Build history of the part. All positions in model axes, mm. A direction names the side the tool comes from. Give positions to 0.01 mm unless a question says otherwise; leave off trailing zeros. Order: outer loops, then holes, each group sorted by start corner. A loop starts at its lowest first (then second) coordinate and runs counter-clockwise, first axis right, second up. Notation, with made-up numbers: (25, 49.25) - (55, 49.25) arc R22 ccw to (55, 79.25) - close; hole circle Ø1 at (10.25, 87). An arc over 180 degrees is marked (long way). Use a Markdown table: item, result. Add a question column.
(1) Flat gauge pins, fed straight in: pin 1 (6 mm diameter, centred on y = -20, z = 23, fed in from +X); pin 2 (4 mm diameter, centred on x = 8.5, z = 6.5, fed in from +Y); pin 3 (12 mm diameter, centred on y = -15.5, z = 14, fed in from +X). Where does each tip first touch, or does it go through?
(2) Which spindle directions (+Z, -Z, +X, -X, +Y, -Y) get a long thin tool onto all of the face, cutting with end or side? Do faces 1 (the face through (17.314, 9.811, 21.731)), 2 (the face through (19, -13, 20.2)), 3 (the face through (-6.092, 27.432, 4.93)). Say none if no direction does.
(3) Slice it at C-C (y = 16.5). Write the cut outline in (x, z), then the cut area to 3 significant figures.
(4) Slice it at B-B (z = 34). Write the cut outline in (x, y).
(5) Slice it at A-A (z = 9). Write the cut outline in (x, y), then the cut area to 3 significant figures.
(6) Slice it at D-D (x = 14). Write the cut outline in (y, z).
(7) Wall check: line 1 (Y direction, x = 0, z = 6); line 2 (Y direction, x = 0, z = 34.75); line 3 (Y direction, x = 0, z = 26). Give the ranges that are in metal, low to high.
(8) Mould opens along Y. For faces 4 (the face through (-28, -21, 2)), 5 (the face through (-2.55, 22, 21)), 6 (the face through (17, -11, 38)), 7 (the face through (0, 24.95, 21)) say: +Y half, -Y half, draft (parallel to the pull), parting line (faces both ways), or undercut.
from build123d import *

# Parameters (mm, degrees)
CUT_EXTRUDE1_DEPTH = 71.512410255
SKETCH3_R          = 1.5
CUT_EXTRUDE2_DEPTH = 20
SKETCH4_W          = 5.1
SKETCH4_H          = 5.05
CUT_EXTRUDE3_DEPTH = 1.8
SKETCH6_R          = 2.55
CUT_EXTRUDE4_DEPTH = 3
SKETCH7_R          = 1.75
CUT_EXTRUDE5_DEPTH = 3
SKETCH8_OUTSIDE_W  = 110.944
SKETCH8_OUTSIDE_H  = 110.944
SKETCH8_OUTSIDE_R  = 35
CUT_EXTRUDE6_DEPTH = 71.512410255


with BuildPart() as part:
    # Sketch1 → Revolve1 (revolve)
    with BuildSketch(Plane(origin=(0, 0, 0), x_dir=(1, 0, 0), z_dir=(0, 1, 0))):
        Polygon((19.9, -38), (19.9, -5), (24.95, -5), (24.95, -10), (28.1, -10), (28.1, 0), (42, 0), (42, -5), (31.25, -5), (31.25, -30), (24.95, -30), (24.95, -38), align=None)
    revolve(axis=Axis((0, 0, 57.825795551), (0, 0, -1)))

    # Sketch2 → Cut-Extrude1 (cut, through all)
    with BuildSketch(Plane.XY.offset(38)):
        Polygon((-22.978540714, 0), (-11.489270357, -19.9), (11.489270357, -19.9), (22.978540714, 0), (11.489270357, 19.9), (-11.489270357, 19.9), align=None)
    extrude(amount=-CUT_EXTRUDE1_DEPTH, mode=Mode.SUBTRACT)

    # Sketch3 → Cut-Extrude2 (cut)
    with BuildSketch(Plane.XY.offset(38)):
        with Locations((0, 22.4)):
            Circle(SKETCH3_R)
        with Locations((19.398969045, -11.2)):
            Circle(SKETCH3_R)
        with Locations((-19.398969045, -11.2)):
            Circle(SKETCH3_R)
    extrude(amount=-CUT_EXTRUDE2_DEPTH, mode=Mode.SUBTRACT)

    # Sketch4 → Cut-Extrude3 (cut)
    with BuildSketch(Plane.XY.offset(22)):
        with Locations((0, 22.425)):
            Rectangle(SKETCH4_W, SKETCH4_H)
        Polygon((18.508905535, -7.74163522), (15.958905535, -12.15836478), (20.332333824, -14.68336478), (22.882333824, -10.26663522), align=None)
        Polygon((-15.958905535, -12.15836478), (-18.508905535, -7.74163522), (-22.882333824, -10.26663522), (-20.332333824, -14.68336478), align=None)
    extrude(amount=-CUT_EXTRUDE3_DEPTH, mode=Mode.SUBTRACT)

    # Sketch6 → Cut-Extrude4 (cut)
    with BuildSketch(Plane(origin=(0, 0, 0), x_dir=(-1, 0, 0), z_dir=(0, 0, -1))):
        with Locations((0, 38)):
            Circle(SKETCH6_R)
        with Locations((38, 0)):
            Circle(SKETCH6_R)
        with Locations((0, -38)):
            Circle(SKETCH6_R)
        with Locations((-38, 0)):
            Circle(SKETCH6_R)
    extrude(amount=-CUT_EXTRUDE4_DEPTH, mode=Mode.SUBTRACT)

    # Sketch7 → Cut-Extrude5 (cut)
    with BuildSketch(Plane(origin=(0, 0, 3), x_dir=(-1, 0, 0), z_dir=(0, 0, -1))):
        with Locations((0, 38)):
            Circle(SKETCH7_R)
        with Locations((38, 0)):
            Circle(SKETCH7_R)
        with Locations((0, -38)):
            Circle(SKETCH7_R)
        with Locations((-38, 0)):
            Circle(SKETCH7_R)
    extrude(amount=-CUT_EXTRUDE5_DEPTH, mode=Mode.SUBTRACT)

    # Sketch8 outside → Cut-Extrude6 (cut, through all)
    with BuildSketch(Plane.XY):
        Rectangle(SKETCH8_OUTSIDE_W, SKETCH8_OUTSIDE_H)
        Circle(SKETCH8_OUTSIDE_R, mode=Mode.SUBTRACT)
    extrude(amount=CUT_EXTRUDE6_DEPTH, mode=Mode.SUBTRACT)


solid = part.part
Solution:
| question | item | result |
|---|---|---|
| 1 | pin 1 | x = 26.22 |
| 1 | pin 2 | y = 34.26 |
| 1 | pin 3 | x = 29.77 |
| 2 | face 1 | +Z, -Z |
| 2 | face 2 | none |
| 2 | face 3 | -Z |
| 3 | outline | (-30.87, 0) - (-22.75, 0) - (-22.75, 10) - (-18.72, 10) - (-18.72, 5) - (-13.45, 5) - (-13.45, 38) - (-18.72, 38) - (-18.72, 30) - (-26.54, 30) - (-26.54, 5) - (-30.87, 5) - close; (13.45, 5) - (18.72, 5) - (18.72, 10) - (22.75, 10) - (22.75, 0) - (30.87, 0) - (30.87, 5) - (26.54, 5) - (26.54, 30) - (18.72, 30) - (18.72, 38) - (13.45, 38) - close |
| 3 | area | 779 mm2 |
| 4 | outline | circle Ø49.9 at (0, 0); hole (-22.98, 0) - (-11.49, -19.9) - (11.49, -19.9) - (22.98, 0) - (11.49, 19.9) - (-11.49, 19.9) - close; hole circle Ø3 at (-19.4, -11.2); hole circle Ø3 at (0, 22.4); hole circle Ø3 at (19.4, -11.2) |
| 5 | outline | circle Ø62.5 at (0, 0); circle Ø49.9 at (0, 0); hole circle Ø56.2 at (0, 0); hole (-22.98, 0) - (-11.49, -19.9) - (11.49, -19.9) - (22.98, 0) - (11.49, 19.9) - (-11.49, 19.9) - close |
| 5 | area | 1,170 mm2 |
| 6 | outline | (-32.08, 0) - (-24.36, 0) - (-24.36, 10) - (-20.65, 10) - (-20.65, 5) - (-15.55, 5) - (-15.55, 38) - (-20.65, 38) - (-20.65, 30) - (-27.94, 30) - (-27.94, 5) - (-32.08, 5) - close; (15.55, 5) - (20.65, 5) - (20.65, 10) - (24.36, 10) - (24.36, 0) - (32.08, 0) - (32.08, 5) - (27.94, 5) - (27.94, 30) - (20.65, 30) - (20.65, 38) - (15.55, 38) - close |
| 7 | line 1 | -31.25 to -28.1, -24.95 to -19.9, 19.9 to 24.95, 28.1 to 31.25 |
| 7 | line 2 | -24.95 to -19.9, 19.9 to 20.9, 23.9 to 24.95 |
| 7 | line 3 | -31.25 to -19.9, 19.9 to 20.9, 23.9 to 31.25 |
| 8 | face 4 | parting line |
| 8 | face 5 | undercut |
| 8 | face 6 | draft |
| 8 | face 7 | undercut |
